Verification items for the finished model (mm, model axes). Face numbers are marked on the shaded views. A direction names the side the tool comes from. Round coordinates to 2 decimals unless told otherwise and drop trailing zeros. Order: outer loops, then holes, each group sorted by start corner. A loop starts at its lowest first (then second) coordinate and runs counter-clockwise, first axis right, second up. Notation, with made-up numbers: (27, 45.25) -> (67, 45.25) arc R16 cw to (67, 57.25) -> close; hole circle Ø9 at (-20.75, 59.25). An arc over 180 degrees is marked (long way). Return JSON: item names as keys, results as strings. Group by question number.
Item 1: Scan lines: probe 1 along Z at (x, y) = (3.5, 4); probe 2 along Z at (x, y) = (-0.5, -2.5); probe 3 along X at (y, z) = (-0.75, 11.5). Record each from-to range of solid material in increasing order. Write a range as from..to.
Item 2: Sectioned sample at C-C on z = 19.25. Record the cut outline in (x, y).
Item 3: Sectioned sample at A-A on x = 3. Record the cut outline in (y, z), plus the area to 3 significant figures.
Item 4: Sectioned sample at B-B on y = -2.75. Record the cut outline in (x, z).
Item 5: Depth check by flat-ended pin: pin 1 Ø3 at (x, z) = (3.5, 12.5) entering from +Y; pin 2 Ø1 at (y, z) = (-2, 9) entering from +X. Enter the tip coordinate at first touch or a pass-through.
Item 6: Access from +Z, -Z, +X, -X, +Y, -Y to the whole of each face (thin tool, end or side, straight path). Record for the marked faces 1 and 2.
Item 7: Sectioned sample at D-D on x = -4. Record the cut outline in (y, z).
```python
from build123d import *

# Parameters (mm, degrees)
F0_R     = 4.75
F1_DEPTH = 20.6
F3_W     = 1.5
F3_H     = 10.714468
F4_DEPTH = 5
F5_W     = 9.5
F5_H     = 9.5
F6_DEPTH = 5


with BuildPart() as f1:
    # F0 (on Top) → F1 (new body)
    with BuildSketch(Plane.XY):
        Circle(F0_R)
    extrude(amount=F1_DEPTH)

    # F3 (on offset) → F4 (cut)
    with BuildSketch(Plane.XY.offset(20.6)):
        Rectangle(F3_W, F3_H)
    extrude(amount=-F4_DEPTH, mode=Mode.SUBTRACT)

    # F5 (on Top) → F6 (join)
    with BuildSketch(Plane.XY):
        Rectangle(F5_W, F5_H)
    extrude(amount=F6_DEPTH)


solid = f1.part
```
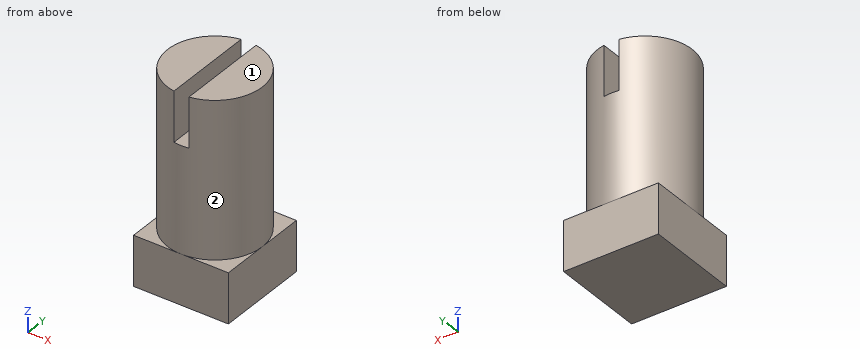
Recorded:
{
 "1": {"probe 1": "0..5", "probe 2": "0..15.6", "probe 3": "-4.69..4.69"},
 "2": {"outline": "(-0.75, -4.69) -> (-0.75, 4.69) arc R4.75 ccw to start; (0.75, -4.69) arc R4.75 ccw to (0.75, 4.69) -> close"},
 "3": {"outline": "(-4.75, 0) -> (4.75, 0) -> (4.75, 5) -> (3.68, 5) -> (3.68, 20.6) -> (-3.68, 20.6) -> (-3.68, 5) -> (-4.75, 5) -> close", "area": "162 mm²"},
 "4": {"outline": "(-4.75, 0) -> (4.75, 0) -> (4.75, 5) -> (3.87, 5) -> (3.87, 20.6) -> (0.75, 20.6) -> (0.75, 15.6) -> (-0.75, 15.6) -> (-0.75, 20.6) -> (-3.87, 20.6) -> (-3.87, 5) -> (-4.75, 5) -> close"},
 "5": {"pin 1": "y = 4.31", "pin 2": "x = 4.51"},
 "6": {"face 1": "+Z, +X, -X, +Y, -Y", "face 2": "+Z"},
 "7": {"outline": "(-4.75, 0) -> (4.75, 0) -> (4.75, 5) -> (2.56, 5) -> (2.56, 20.6) -> (-2.56, 20.6) -> (-2.56, 5) -> (-4.75, 5) -> close"}
}
